from build123d import *

# Parameters (mm, degrees)
SKETCH1_R                = 2.5
BOSS_EXTRUDE1_DEPTH      = 1
SKETCH2_R                = 3.5
SKETCH2_R_2              = 3
BOSS_EXTRUDE2_DEPTH      = 1.5
SKETCH3_W                = 10
SKETCH3_H                = 10
BOSS_EXTRUDE3_DEPTH      = 10
BOSS_EXTRUDE4_DEPTH      = 35
BOSS_EXTRUDE4_DEPTH_BACK = 45
SKETCH4_W                = 5
SKETCH4_H                = 5
BOSS_EXTRUDE5_DEPTH      = 2
BOSS_EXTRUDE5_DEPTH_BACK = 110
SKETCH5_W                = 5
SKETCH5_H                = 5
CUT_EXTRUDE4_START       = -10
SKETCH6_W                = 9.9
SKETCH6_H                = 10
SKETCH6_R                = 2.5
CUT_EXTRUDE4_DEPTH       = 1
SKETCH6_3_R              = 2.5
SKETCH6_3_W              = 0.1
SKETCH6_3_H              = 10
CUT_EXTRUDE5_DEPTH       = 3


with BuildPart() as part:
    # Sketch1 → Boss-Extrude1 (new body)
    with BuildSketch(Plane(origin=(0, 0, 0), x_dir=(1, 0, 0), z_dir=(0, 1, 0))):
        with BuildLine():
            Line((-54, -40), (54, -40))
            ThreePointArc((54, -40), (58.242640687, -38.242640687), (60, -34))
            Line((60, -34), (60, 34))
            ThreePointArc((60, 34), (58.242640687, 38.242640687), (54, 40))
            Line((54, 40), (-54, 40))
            ThreePointArc((-54, 40), (-58.242640687, 38.242640687), (-60, 34))
            Line((-60, 34), (-60, -34))
            ThreePointArc((-60, -34), (-58.242640687, -38.242640687), (-54, -40))
        make_face()
        with Locations(Location((0, 31.25, 0), (0, 0, 270))):
            Circle(SKETCH1_R, mode=Mode.SUBTRACT)
        with Locations(Location((0, -32.75, 0), (0, 0, 270))):
            Circle(SKETCH1_R, mode=Mode.SUBTRACT)
    extrude(amount=BOSS_EXTRUDE1_DEPTH)

    # Sketch2 → Boss-Extrude2 (add)
    with BuildSketch(Plane.XZ):
        with Locations(Location((-54, 34, 0), (0, 0, 90))):
            Circle(SKETCH2_R)
        with Locations(Location((-54, 0, 0), (0, 0, 90))):
            Circle(SKETCH2_R_2)
        with Locations(Location((-54, -34, 0), (0, 0, 90))):
            Circle(SKETCH2_R)
        with Locations(Location((54, 34, 0), (0, 0, 90))):
            Circle(SKETCH2_R)
        with Locations(Location((54, -34, 0), (0, 0, 90))):
            Circle(SKETCH2_R)
        with Locations(Location((54, 0, 0), (0, 0, 90))):
            Circle(SKETCH2_R_2)
    extrude(amount=BOSS_EXTRUDE2_DEPTH)

    # Sketch3 → Boss-Extrude3 (add)
    with BuildSketch(Plane(origin=(0, 1, 0), x_dir=(1, 0, 0), z_dir=(0, 1, 0))):
        with Locations((54, 0)):
            Rectangle(SKETCH3_W, SKETCH3_H)
        with Locations((44, 0)):
            Rectangle(SKETCH3_W, SKETCH3_H)
        with Locations((-53, 0)):
            Rectangle(SKETCH3_W, SKETCH3_H)
    extrude(amount=BOSS_EXTRUDE3_DEPTH)

    # Sketch4 → Boss-Extrude4 (add, two sides: drawn at the far end of the back side and taken through both)
    with BuildSketch(Plane.XY.offset(5).offset(-BOSS_EXTRUDE4_DEPTH_BACK)):
        with Locations((-53, 6)):
            Rectangle(SKETCH4_W, SKETCH4_H)
    extrude(amount=BOSS_EXTRUDE4_DEPTH + BOSS_EXTRUDE4_DEPTH_BACK)

    # Sketch5 → Boss-Extrude5 (add, two sides: drawn at the far end of the back side and taken through both)
    with BuildSketch(Plane(origin=(59, 0, 0), x_dir=(0, 0, -1), z_dir=(1, 0, 0)).offset(-BOSS_EXTRUDE5_DEPTH_BACK)):
        with Locations((0, 6)):
            Rectangle(SKETCH5_W, SKETCH5_H)
    extrude(amount=BOSS_EXTRUDE5_DEPTH + BOSS_EXTRUDE5_DEPTH_BACK)

    # Sketch6 → Cut-Extrude4 (cut)
    # profile 1 of 2: a face of its own
    with BuildSketch(Plane(origin=(0, 11, 0), x_dir=(1, 0, 0), z_dir=(0, 1, 0)).offset(CUT_EXTRUDE4_START)):
        with Locations((43.95, 0)):
            Rectangle(SKETCH6_W, SKETCH6_H)
        with Locations((44, 0)):
            Circle(SKETCH6_R, mode=Mode.SUBTRACT)
    # profile 2 of 2: a face of its own
    with BuildSketch(Plane(origin=(0, 11, 0), x_dir=(1, 0, 0), z_dir=(0, 1, 0)).offset(CUT_EXTRUDE4_START)):
        with Locations((44, 0)):
            Circle(SKETCH6_R)
    extrude(amount=CUT_EXTRUDE4_DEPTH, mode=Mode.SUBTRACT)

    # Sketch6<3> → Cut-Extrude5 (cut)
    with BuildSketch(Plane(origin=(0, 11, 0), x_dir=(1, 0, 0), z_dir=(0, 1, 0))):
        with Locations(Location((44, 0, 0), (0, 0, 270))):
            Circle(SKETCH6_3_R)
        with Locations((48.95, 0)):
            Rectangle(SKETCH6_3_W, SKETCH6_3_H)
    extrude(amount=-CUT_EXTRUDE5_DEPTH, mode=Mode.SUBTRACT)


solid = part.part
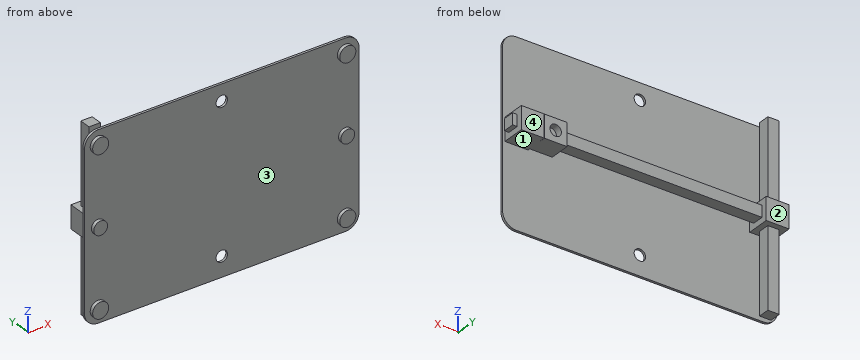
CAD build for the part. Positions are in the model's coordinates, mm. Face numbers are marked on the shaded views. A direction names the side the tool comes from. Round coordinates to 2 decimals unless told otherwise and drop trailing zeros. Write each loop counter-clockwise with the first axis right and the second up, starting at its lowest first coordinate (ties: lowest second). Pieces come first, ordered by that corner, then holes. Notation, with made-up numbers: M 2.25,83.25 L 39.25,83.25 A19 cw 39.25,97.25 Z; hole C -5,72 d8. An arc over 180 degrees is marked long. Put each result on its own line as item: value. Start each with the question number.
1) Saw through at A-A, the plane y = 9.75. Write the cut outline in (x, z).
2) Pull direction X, two halves, no side cores. Call the marked faces 3 and 4: pulls with the +X half, pulls with the -X half, needs draft (parallel to the pull), parting line crosses it, or undercut.
3) Pin check, flat tips, straight feed: pin 1 Ø1.5 at (x, z) = (-52, 14) entering from +Y; pin 2 Ø6 at (x, z) = (29.5, 11.5) entering from -Y; pin 3 Ø0.9 at (y, z) = (9, -1.5) entering from +X. Stop position of each tip, or through.
4) Saw through at D-D, the plane x = 0. Write the cut outline in (y, z), and give its area (3 significant figures).
5) Saw through at C-C, the plane z = 32.75. Write the cut outline in (x, y), and give its area (3 significant figures).
6) 3-axis set-ups, long thin cutter, end or side, ignore diameter. For the marked faces 1 and 2: which of +Z, -Z, +X, -X, +Y, -Y reach the whole face in a straight line?
7) Drill centre lines: probe 1 along X at (y, z) = (0.25, 32.75); probe 2 along X at (y, z) = (7.75, 20); probe 3 along Y at (x, z) = (39.5, 0). Where is each one in solid material? Low to high. Write a range as [from, to].
8) Saw through at B-B, the plane x = -29. Write the cut outline in (y, z).
Resolved:
1. outline: M -58,-5 L -48,-5 L -48,5 L -58,5 Z; M 39,-5 L 48.9,-5 L 48.9,5 L 39,5 Z; M 49,-5 L 59,-5 L 59,5 L 49,5 Z; hole C 44,0 d5
2. face 3: undercut
2. face 4: needs draft
3. pin 1: y = 8.5
3. pin 2: y = 0
3. pin 3: x = 59
4. outline: M 0,-40 L 1,-40 L 1,-33.75 L 0,-33.75 Z; M 0,-28.75 L 1,-28.75 L 1,30.25 L 0,30.25 Z; M 0,35.25 L 1,35.25 L 1,40 L 0,40 Z; M 3.5,-2.5 L 8.5,-2.5 L 8.5,2.5 L 3.5,2.5 Z
4. area: 95.0 mm²
5. outline: M -60,0 L -57.27,0 L -57.27,-1.5 L -50.73,-1.5 L -50.73,0 L -2.5,0 L -2.5,1 L -60,1 Z; M -55.5,3.5 L -50.5,3.5 L -50.5,8.5 L -55.5,8.5 Z; M 2.5,0 L 50.73,0 L 50.73,-1.5 L 57.27,-1.5 L 57.27,0 L 60,0 L 60,1 L 2.5,1 Z
5. area: 160 mm²
6. face 1: -Z, +X, +Y
6. face 2: +Z, -Z, +X, -X, +Y
7. probe 1: [-60, -2.5], [2.5, 60]
7. probe 2: [-55.5, -50.5]
7. probe 3: [0, 1], [2, 11]
8. outline: M 0,-40 L 1,-40 L 1,40 L 0,40 Z; M 3.5,-2.5 L 8.5,-2.5 L 8.5,2.5 L 3.5,2.5 Z
